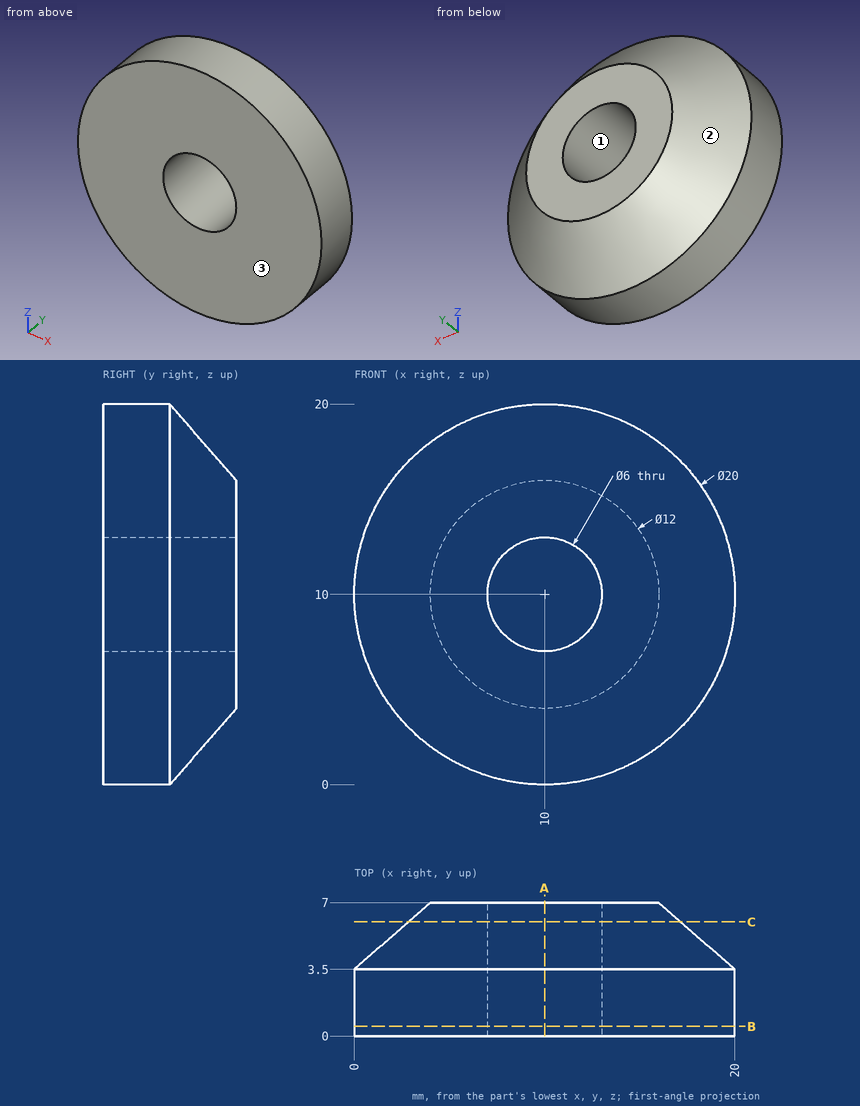
Can you work these out from the drawing? Everything is in mm from the part's minimum corner. Round coordinates to 2 decimals unless told otherwise and drop trailing zeros. Write each loop counter-clockwise with the first axis right and the second up, starting at its lowest first coordinate (ties: lowest second). Pieces come first, ordered by that corner, then holes. Notation, with made-up numbers: (7.25, -32.5) - (19.25, -32.5) arc R15 ccw to (19.25, -26.5) - close; hole circle Ø8 at (22, 80). An arc over 180 degrees is marked (long way). Write each question's results on one line, items separated by ' | '. Start each with the question number.
1) We'd pull the mould along X, two halves only. Please class the marked faces 1, 2 and 3: released by +X, released by -X, zero draft, split by the parting line, or undercut.
2) Please list where these lines run through material, in increasing order: line 1 (Z direction, x = 10, y = 1.5); line 2 (X direction, y = 1.5, z = 9.5); line 3 (X direction, y = 6.75, z = 11).
3) Suppose I cut it at C-C (y = 6). List the corners of the cut face in (x, z) for me.
4) Suppose I cut it at A-A (x = 10). List the corners of the cut face in (y, z) for me.
5) Suppose I cut it at B-B (y = 0.5). List the corners of the cut face in (x, z) for me, and give its area (3 significant figures).
6) For pin 1 Ø1 at (y, z) = (1.5, 16) entering from +X; pin 2 Ø1.5 at (y, z) = (1.5, 15.5) entering from -X, each with a flat end and sliding along its axis, tell me the tip position at first contact or that it passes through.
Here are the results:
1) face 1: undercut | face 2: split by the parting line | face 3: zero draft
2) line 1: z = 0 to 7, 13 to 20 | line 2: x = 0.01 to 7.04, 12.96 to 19.99 | line 3: x = 3.79 to 7.17, 12.83 to 16.21
3) outline: circle Ø14.29 at (10, 10); hole circle Ø6 at (10, 10)
4) outline: (0, 0) - (3.5, 0) - (7, 4) - (7, 7) - (0, 7) - close; (0, 13) - (7, 13) - (7, 16) - (3.5, 20) - (0, 20) - close
5) outline: circle Ø20 at (10, 10); hole circle Ø6 at (10, 10) | area: 286 mm2
6) pin 1: stops at x = 18.35 | pin 2: stops at x = 1.2
